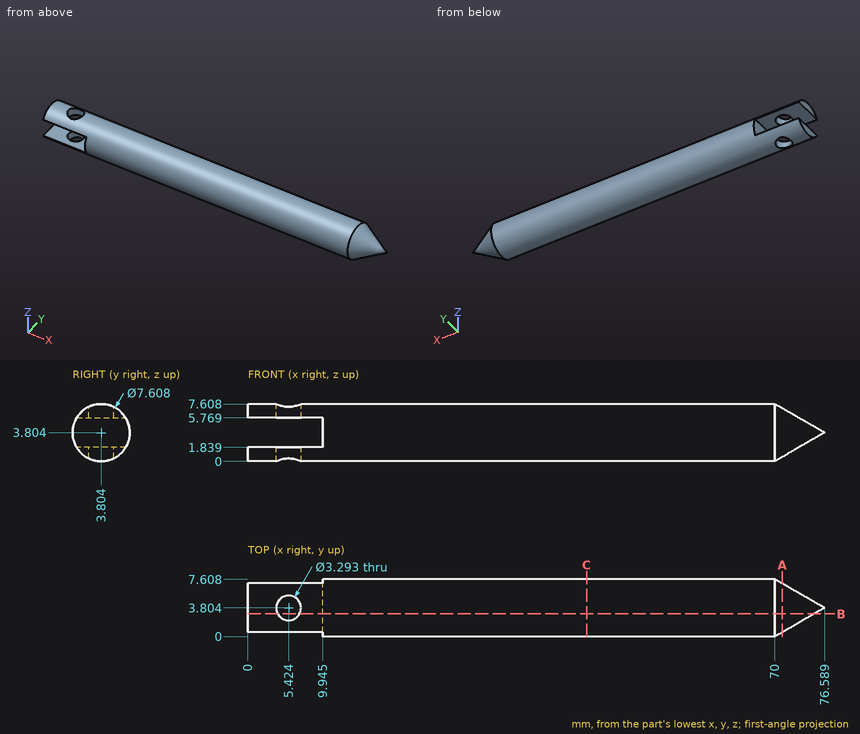
The drawing under review shows one solid part. Ordinate dimensions are in mm from its lowest x, y, z. Coordinates: 2 decimals unless noted, no trailing zeros. Write each loop counter-clockwise with the first axis right and the second up, starting at its lowest first coordinate (ties: lowest second). Pieces come first, ordered by that corner, then holes. Notation, with made-up numbers: (-34.75, 84) - (-1.75, 84) arc R33 ccw to (-1.75, 114) - close; hole circle Ø2 at (0.25, 24.25). An arc over 180 degrees is marked (long way). Answer as CSV lines item,"result".
(1) We need section B-B (y = 3). Count the separate pieces of the cut face and the enclosed holes in it, plus the area to 3 significant figures.
Data:
separate pieces,"3"
enclosed holes,"0"
area,"493 mm2"
(2) Clearance check with flat-ended pins moving along their axes: pin 1 Ø2 at (x, y) = (2.5, 5) entering from +Z; pin 2 Ø3 at (x, y) = (5.42, 3.8) entering from -Z; pin 3 Ø2 at (x, z) = (14, 2) entering from -Y; pin 4 Ø4 at (x, y) = (19.5, 1.5) entering from -Z. State where each tip first meets the part, or that it passes through.
Data:
pin 1,"stops at z = 7.6"
pin 2,"passes through"
pin 3,"stops at y = 0.09"
pin 4,"stops at z = 0.01"
(3) We need section A-A (x = 71). Give the boundary of the cut face in (y, z).
Data:
outline,"circle Ø6.45 at (3.8, 3.8)"
(4) For line 1 along Z through (x, y) = (65, 3.5); line 2 along Y through (x, z) = (19, 4) (1 decimal); line 3 along Z through (x, y) = (5.5, 2) (1 decimal), list the stretches that pass through material, from the lowest coordinate up. Write a range as [from, to].
Data:
line 1,"z = [0.01, 7.6]"
line 2,"y = [0, 7.6]"
line 3,"z = [0.5, 1.8], [5.8, 7.2]"
(5) We need section C-C (x = 45). Give the boundary of the cut face in (y, z).
Data:
outline,"circle Ø7.61 at (3.8, 3.8)"
